Verification items for the finished model (mm, model axes). A direction names the side the tool comes from. Give positions to 0.01 mm unless a question says otherwise; leave off trailing zeros. Loops run counter-clockwise (first coordinate to the right, second up) from the corner with the lowest first, then second, coordinate; pieces in that order, holes last. Notation, with made-up numbers: M 38,75.5 L 63,75.5 A14 ccw 63,91.5 Z; hole C 28,68 d7. An arc over 180 degrees is marked long. Use a Markdown table: item, result.
from build123d import *

# Parameters (mm, degrees)
ESQUISSE1_W             = 12.7
ESQUISSE1_H             = 12.7
BOSS_EXTRU_1_DEPTH      = 4.7625
ESQUISSE2_R             = 2.6
ENL_V_MAT_EXTRU_1_DEPTH = 14.090860361
ESQUISSE4_W             = 9.525
ESQUISSE4_H             = 12.7
BOSS_EXTRU_3_DEPTH      = 51.8414
ESQUISSE5_R             = 2.6797
ENL_V_MAT_EXTRU_2_DEPTH = 60.306721027
ESQUISSE6_W             = 9.525
ESQUISSE6_H             = 3.175
ENL_V_MAT_EXTRU_3_DEPTH = 60.751237981
ESQUISSE7_W             = 9.525
ESQUISSE7_H             = 12.7
BOSS_EXTRU_4_DEPTH      = 34.925
BOSS_EXTRU_5_DEPTH      = 12.7
ESQUISSE9_R             = 2.6
ENL_V_MAT_EXTRU_4_DEPTH = 90.183031598


with BuildPart() as part:
    # Esquisse1 → Boss.-Extru.1 (new, symmetric)
    with BuildSketch(Plane.XY):
        Rectangle(ESQUISSE1_W, ESQUISSE1_H)
    extrude(amount=BOSS_EXTRU_1_DEPTH, both=True)

    # Esquisse2 → Enlèv. mat.-Extru.1 (cut, through all)
    with BuildSketch(Plane.XY.offset(4.7625)):
        Circle(ESQUISSE2_R)
    extrude(amount=-ENL_V_MAT_EXTRU_1_DEPTH, mode=Mode.SUBTRACT)

    # Esquisse4 → Boss.-Extru.3 (add)
    with BuildSketch(Plane(origin=(6.35, 0, 0), x_dir=(0, 0, -1), z_dir=(1, 0, 0))):
        Rectangle(ESQUISSE4_W, ESQUISSE4_H)
    extrude(amount=BOSS_EXTRU_3_DEPTH)

    # Esquisse5 → Enlèv. mat.-Extru.2 (cut, through all)
    with BuildSketch(Plane.XY.offset(4.7625)):
        with Locations((51.8414, 0)):
            Circle(ESQUISSE5_R)
    extrude(amount=-ENL_V_MAT_EXTRU_2_DEPTH, mode=Mode.SUBTRACT)

    # Esquisse6 → Enlèv. mat.-Extru.3 (cut, through all)
    with BuildSketch(Plane(origin=(0, 6.35, 0), x_dir=(1, 0, 0), z_dir=(0, 1, 0))):
        with Locations((53.4289, 0)):
            Rectangle(ESQUISSE6_W, ESQUISSE6_H)
    extrude(amount=-ENL_V_MAT_EXTRU_3_DEPTH, mode=Mode.SUBTRACT)

    # Esquisse7 → Boss.-Extru.4 (add)
    with BuildSketch(Plane.ZY.offset(6.35)):
        Rectangle(ESQUISSE7_W, ESQUISSE7_H)
    extrude(amount=BOSS_EXTRU_4_DEPTH)

    # Esquisse8 → Boss.-Extru.5 (add)
    with BuildSketch(Plane(origin=(0, 6.35, 0), x_dir=(1, 0, 0), z_dir=(0, 1, 0))):
        Polygon((-37.057243879, 4.7625), (-57.694743879, 25.4), (-73.025, 25.4), (-73.025, 19.05), (-60.325, 19.05), (-41.275, 0), (-60.325, -19.05), (-73.025, -19.05), (-73.025, -25.4), (-57.694743879, -25.4), (-37.057243879, -4.7625), align=None)
    extrude(amount=-BOSS_EXTRU_5_DEPTH)

    # Esquisse9 → Enlèv. mat.-Extru.4 (cut, through all)
    with BuildSketch(Plane.XY.offset(25.4)):
        with Locations((-65.405, 0)):
            Circle(ESQUISSE9_R)
    extrude(amount=-ENL_V_MAT_EXTRU_4_DEPTH, mode=Mode.SUBTRACT)


solid = part.part
(1) Gauge pin test, flat ends, axial feed: P1, Ø5, axis at x = 53, y = -1, coming from the +Z side; P2, Ø7, axis at x = 51.84, y = 0, coming from the -Z side; P3, Ø1.6, axis at y = 1, z = -0.5, coming from the +X side; P4, Ø3, axis at x = -65.405, y = 0, coming from the +Z side. Record the tip position at first contact, or that the pin passes through.
Results below:
| item | result |
|---|---|
| P1 | z = 4.76 |
| P2 | z = -4.76 |
| P3 | x = 48.67 |
| P4 | through |
(2) Draft check along Y on faces 4 (the flat face through (-13, 6.35, 2)), 5 (the cylindrical face through (-62.925, 0.781, 22.269)), 6 (the flat face through (-50.933, 0.089, -9.658)), 7 (the cylindrical face through (-0.338, 2.578, 0.067)). Enter one of: +Y half, -Y half, draft (parallel to the pull), parting line (faces both ways), or undercut.
Results below:
| item | result |
|---|---|
| face 4 | +Y half |
| face 5 | undercut |
| face 6 | draft |
| face 7 | undercut |
(3) Cross-section at C-C on x = -55. Record the cut outline in (y, z) (3 decimals).
Results below:
| item | result |
|---|---|
| outline | M -6.35,-22.705 L 6.35,-22.705 L 6.35,-13.725 L -6.35,-13.725 Z; M -6.35,13.725 L 6.35,13.725 L 6.35,22.705 L -6.35,22.705 Z |
(4) Cross-section at B-B on y = 0. State how many separate pieces and enclosed holes the cut face has, then the cut area to 3 significant figures.
Results below:
| item | result |
|---|---|
| separate pieces | 6 |
| enclosed holes | 0 |
| area | 1,280 mm^2 |
(5) Cross-section at A-A on x = 0. Record the cut outline in (y, z).
Results below:
| item | result |
|---|---|
| outline | M -6.35,-4.76 L -2.6,-4.76 L -2.6,4.76 L -6.35,4.76 Z; M 2.6,-4.76 L 6.35,-4.76 L 6.35,4.76 L 2.6,4.76 Z |
(6) Material ranges on line 1 (Y direction, x = 0, z = 1); line 2 (Z direction, x = 50.5, y = -3.75); line 3 (Z direction, x = -33.5, y = 4), recorded low to high.
Results below:
| item | result |
|---|---|
| line 1 | -6.35 to -2.6, 2.6 to 6.35 |
| line 2 | -4.76 to -1.59, 1.59 to 4.76 |
| line 3 | -4.76 to 4.76 |
(7) Set-up check for faces 1 (the flat face through (11, 0, -4.762)), 2 (the flat face through (-68.2, 0.1, -19.05)), 3 (the flat face through (54.4, -1.3, 1.588)): record each of +Z, -Z, +X, -X, +Y, -Y from which the full face is reachable in a straight line by a thin tool's end or side.
Results below:
| item | result |
|---|---|
| face 1 | -Z, +X, +Y, -Y |
| face 2 | -X, +Y, -Y |
| face 3 | +X, +Y, -Y |
(8) Cross-section at D-D on z = -3.5. Record the cut outline in (x, y) (3 decimals).
Results below:
| item | result |
|---|---|
| outline | M -44.775,-6.35 L 58.191,-6.35 L 58.191,6.35 L -44.775,6.35 Z; hole C 0,0 d5.2; hole C 51.841,0 d5.359 |
